from build123d import *

# Parameters (mm, degrees)
BOSS_EXTRUDE1_DEPTH = 15
FILLET1_R           = 5
SKETCH4_W           = 6.2
SKETCH4_H           = 6.2
CUT_EXTRUDE1_DEPTH  = 3.25
SKETCH5_W           = 6.2
SKETCH5_H           = 6.2
CUT_EXTRUDE2_DEPTH  = 3.25
SKETCH8_W           = 6.2
SKETCH8_H           = 6.2
CUT_EXTRUDE3_DEPTH  = 10
SKETCH9_W           = 6.2
SKETCH9_H           = 6.158762439
CUT_EXTRUDE4_DEPTH  = 8
SKETCH10_W          = 6.2
SKETCH10_H          = 6.244686175
CUT_EXTRUDE6_DEPTH  = 20
SKETCH11_R          = 1.5
CUT_EXTRUDE7_DEPTH  = 36


with BuildPart() as part:
    # Sketch2 → Boss-Extrude1 (new body)
    with BuildSketch(Plane.XY):
        Polygon((29.5, -24.5), (29.5, 0.5), (17.5, 12.5), (-0.5, 12.5), (-0.5, -9.5), (15.5, -24.5), align=None)
    extrude(amount=BOSS_EXTRUDE1_DEPTH)

    # Fillet1
    fillet1_edges = [part.edges().sort_by_distance(p)[0] for p in [
        (15.5, -24.5, 7.5),
        (17.5, 12.5, 7.5),
        (23.5, 6.5, 15),
        (8.5, 12.5, 15),
        (7.5, -17, 15),
        (22.5, -24.5, 15),
        (7.5, -17, 0),
        (8.5, 12.5, 0),
        (23.5, 6.5, 0),
        (22.5, -24.5, 0),
    ]]
    fillet(fillet1_edges, radius=FILLET1_R)

    # Sketch4 → Cut-Extrude1 (cut)
    with BuildSketch(Plane(origin=(29.5, 0, 0), x_dir=(0, 0, -1), z_dir=(1, 0, 0))):
        with Locations((-6, -17.6)):
            Rectangle(SKETCH4_W, SKETCH4_H)
        with Locations((-6, -6.4)):
            Rectangle(SKETCH4_W, SKETCH4_H)
    extrude(amount=-CUT_EXTRUDE1_DEPTH, mode=Mode.SUBTRACT)

    # Sketch5 → Cut-Extrude2 (cut)
    with BuildSketch(Plane.ZY.offset(0.5)):
        with Locations((7.5, 1.5)):
            Rectangle(SKETCH5_W, SKETCH5_H)
    extrude(amount=-CUT_EXTRUDE2_DEPTH, mode=Mode.SUBTRACT)

    # Sketch8 → Cut-Extrude3 (cut)
    with BuildSketch(Plane.ZY.offset(-2.75)):
        with Locations((7.5, 1.5)):
            Rectangle(SKETCH8_W, SKETCH8_H)
    extrude(amount=-CUT_EXTRUDE3_DEPTH, mode=Mode.SUBTRACT)

    # Sketch9 → Cut-Extrude4 (cut)
    with BuildSketch(Plane(origin=(0, -1.6, 0), x_dir=(1, 0, 0), z_dir=(0, 1, 0))):
        with Locations((9.626788027, -7.520618781)):
            Rectangle(SKETCH9_W, SKETCH9_H)
    extrude(amount=-CUT_EXTRUDE4_DEPTH, mode=Mode.SUBTRACT)

    # Sketch10 → Cut-Extrude6 (cut)
    with BuildSketch(Plane(origin=(26.25, 0, 0), x_dir=(0, 0, -1), z_dir=(1, 0, 0))):
        with Locations((-6, -6.377656912)):
            Rectangle(SKETCH10_W, SKETCH10_H)
    extrude(amount=-CUT_EXTRUDE6_DEPTH, mode=Mode.SUBTRACT)

    # Sketch11 → Cut-Extrude7 (cut)
    with BuildSketch(Plane(origin=(29.5, 0, 0), x_dir=(0, 0, -1), z_dir=(1, 0, 0))):
        with Locations((-12.118468993, -7.263784025)):
            Circle(SKETCH11_R)
    extrude(amount=-CUT_EXTRUDE7_DEPTH, mode=Mode.SUBTRACT)


solid = part.part
Geometry check sheet. Reference: the model listing, model coordinates, mm. A direction names the side the tool comes from. Give positions to 0.01 mm unless a question says otherwise; leave off trailing zeros. Order: outer loops, then holes, each group sorted by start corner. A loop starts at its lowest first (then second) coordinate and runs counter-clockwise, first axis right, second up.
1) Tool access check on faces 4 (the flat face through (6.527, -4, 10)), 5 (the flat face through (28, -18, 9.1)), 6 (the cylindrical face through (14.71, -7.838, 10.733)), 7 (the flat face through (3, -1.6, 7)), 8 (the flat face through (29.5, -12, 7)). Record the directions out of +Z, -Z, +X, -X, +Y, -Y that give a thin tool (end or side, any length) a straight path to the whole face; none if there is none.
Results are:
face 4: none
face 5: +X
face 6: +X, -X
face 7: -X
face 8: +Z, -Z, +X, +Y, -Y
2) Draft check along Y on faces 1 (the flat face through (24, 6, 7)), 2 (the cylindrical face through (6.17, -13.799, 1.504)), 3 (the flat face through (10, -9.6, 7)). Enter one of: released by +Y, released by -Y, zero draft, split by the parting line, or undercut.
Results are:
face 1: released by +Y
face 2: released by -Y
face 3: undercut
3) Cross-section at B-B (z = 1.5). Record the boundary of the cut face in (x, y).
Results are:
outline: (-0.5, -7.54) - (15.04, -22.1) arc R3.57 ccw to (17.48, -23.07) - (29.5, -23.07) - (29.5, -1.52) - (17.95, 10.02) arc R3.57 ccw to (15.43, 11.07) - (-0.5, 11.07) - close
4) Cross-section at C-C (x = 10.5). Give the number of separate pieces and of enclosed holes in the cut face, then the cut area to 3 significant figures.
Results are:
separate pieces: 1
enclosed holes: 2
area: 355 mm2
5) Gauge pin test, flat ends, axial feed: pin 1 (6 mm diameter, centred on x = 23.5, z = 5, fed in from +Y); pin 2 (3 mm diameter, centred on x = 7, z = 9, fed in from -Y); pin 3 (1.9 mm diameter, centred on y = 2, z = 7.5, fed in from -X). Record the tip position at first contact, or that the pin passes through.
Results are:
pin 1: stops at y = 9.5
pin 2: stops at y = -17.94
pin 3: stops at x = 12.75
6) Material ranges on probe 1 along Z at (x, y) = (7, -4); probe 2 along Z at (x, y) = (2.5, 0.5); probe 3 along X at (y, z) = (-5.5, 6.5), recorded low to high.
Results are:
probe 1: z = 0 to 2.9, 10.6 to 15
probe 2: z = 0 to 4.4, 10.6 to 15
probe 3: x = -0.5 to 6.25
